Geometry: see drawing. Coordinates: mm, zero at the bounding-box minimum. Coordinates: 2 decimals unless noted, no trailing zeros. Order: outer loops, then holes, each group sorted by start corner. A loop starts at its lowest first (then second) coordinate and runs counter-clockwise, first axis right, second up. Notation, with made-up numbers: M -31.5,30.5 L 6.5,30.5 A24 cw 6.5,55.5 Z; hole C 17.25,-17 d6. An arc over 180 degrees is marked long. Answer in a Markdown table with one row per item.
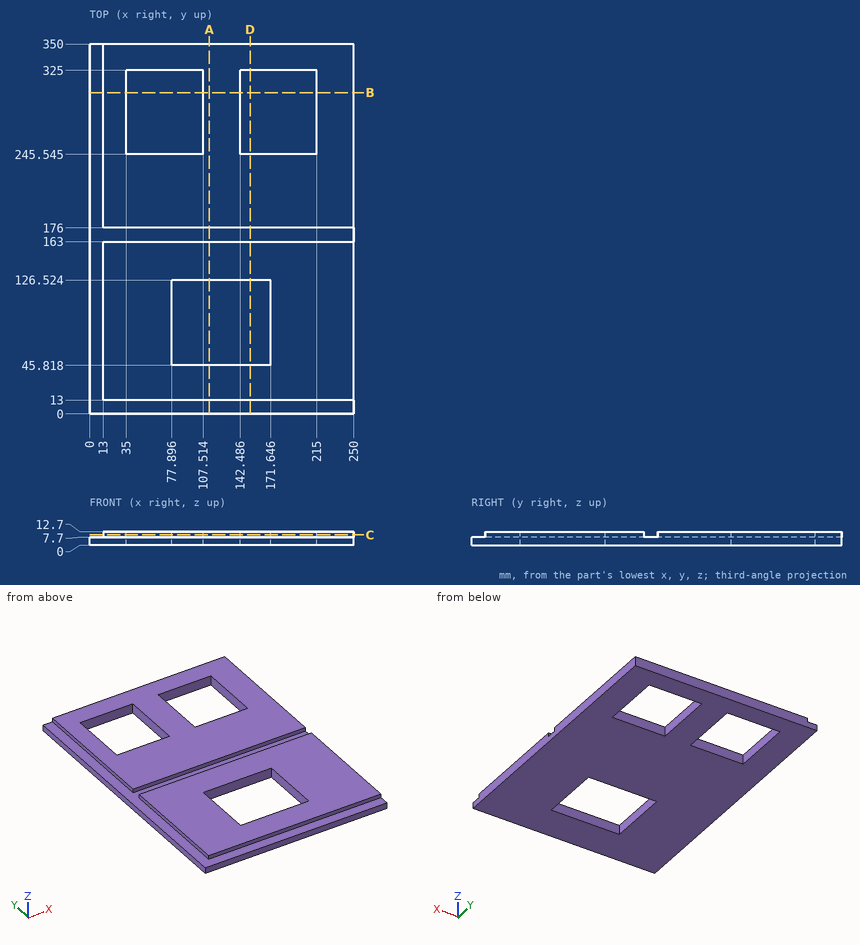
1) Cut plane B-B, the plane y = 304. Output: boundary loops of the cut face in (x, z) (1 decimal), and give its area (3 significant figures).
Resolved:
| item | result |
|---|---|
| outline | M 0,0 L 35,0 L 35,12.7 L 13,12.7 L 13,7.7 L 0,7.7 Z; M 107.5,0 L 142.5,0 L 142.5,12.7 L 107.5,12.7 Z; M 215,0 L 250,0 L 250,12.7 L 215,12.7 Z |
| area | 1,270 mm2 |
2) Cut plane A-A, the plane x = 113.5. Output: boundary loops of the cut face in (y, z) (1 decimal), and give its area (3 significant figures).
Resolved:
| item | result |
|---|---|
| outline | M 0,0 L 45.8,0 L 45.8,12.7 L 13,12.7 L 13,7.7 L 0,7.7 Z; M 126.5,0 L 350,0 L 350,12.7 L 176,12.7 L 176,7.7 L 163,7.7 L 163,12.7 L 126.5,12.7 Z |
| area | 3,290 mm2 |
3) Cut plane C-C, the plane z = 9.75. Output: boundary loops of the cut face in (x, y) (1 decimal).
Resolved:
| item | result |
|---|---|
| outline | M 13,13 L 250,13 L 250,163 L 13,163 Z; M 13,176 L 250,176 L 250,350 L 13,350 Z; hole M 35,245.5 L 107.5,245.5 L 107.5,325 L 35,325 Z; hole M 77.9,45.8 L 171.6,45.8 L 171.6,126.5 L 77.9,126.5 Z; hole M 142.5,245.5 L 215,245.5 L 215,325 L 142.5,325 Z |
4) Material intervals for probe 1 along X at (y, z) = (288.5, 10) (1 decimal); probe 2 along Y at (x, z) = (97.5, 9.5) (1 decimal); probe 3 along X at (y, z) = (272.5, 3.5) (1 decimal), sorted ascending.
Resolved:
| item | result |
|---|---|
| probe 1 | x = 13 to 35, 107.5 to 142.5, 215 to 250 |
| probe 2 | y = 13 to 45.8, 126.5 to 163, 176 to 245.5, 325 to 350 |
| probe 3 | x = 0 to 35, 107.5 to 142.5, 215 to 250 |
5) Contact query for flat-ended pins moving along their axis: pin 1 (6 mm diameter, centred on x = 196, z = 6.5, fed in from -Y); pin 2 (1.5 mm diameter, centred on x = 186, z = 10, fed in from -Y); pin 3 (4 mm diameter, centred on y = 100, z = 10.5, fed in from -X). Output: stop coordinate, or through.
Resolved:
| item | result |
|---|---|
| pin 1 | stops at y = 0 |
| pin 2 | stops at y = 13 |
| pin 3 | stops at x = 13 |
6) Cut plane D-D, the plane x = 152. Output: boundary loops of the cut face in (y, z) (1 decimal), and give its area (3 significant figures).
Resolved:
| item | result |
|---|---|
| outline | M 0,0 L 45.8,0 L 45.8,12.7 L 13,12.7 L 13,7.7 L 0,7.7 Z; M 126.5,0 L 245.5,0 L 245.5,12.7 L 176,12.7 L 176,7.7 L 163,7.7 L 163,12.7 L 126.5,12.7 Z; M 325,0 L 350,0 L 350,12.7 L 325,12.7 Z |
| area | 2,280 mm2 |
